Autodesk Inventor part; units mm, degrees
ref_plane "YZ Plane" through (0, 0, 0) normal (1, 0, 0) x (0, 1, 0)
ref_plane "XZ Plane" through (0, 0, 0) normal (0, 1, 0) x (-1, 0, 0)
ref_plane "XY Plane" through (0, 0, 0) normal (0, 0, 1) x (1, 0, 0)
sketch "Sketch1" plane through (0, 0, 0) normal (0, 1, 0) x (-1, 0, 0)
  line L0 (8.5, -37.5) -> (8.5, 37.5) construction
  line L1 (-8.5, 37.5) -> (-8.5, -37.5) construction
  line L2 (15.5, 33) -> (15.5, -33)
  line L3 (-15.5, -33) -> (-15.5, 33) construction
  line L4 (15.5, -33) -> (-15.5, -33)
  line L5 (-8.5, -37.5) -> (8.5, -37.5) construction
  circle A0 centre (8.5, -37.5) radius 2.25
  line L6 (0, -37.5) -> (-8.5, -37.5) construction
  circle A1 centre (-8.5, -37.5) radius 2.25
  line L7 (-15.5, 33) -> (15.5, 33)
  circle A2 centre (-8.5, 37.5) radius 2.25
  line L8 (8.5, 37.5) -> (-8.5, 37.5) construction
  circle A3 centre (8.5, 37.5) radius 2.25
  line L9 (-15.5, -33) -> (15.5, 33) construction
  line L10 (0, 33) -> (0, 19.5) construction
  line L11 (0, 0) -> (15.5, 0) construction
  line L12 (0, 19.5) -> (-39.9, 19.5) construction
  line L13 (-54.9, -40.5) -> (-24.9, -40.5) construction
  circle A4 centre (-54.9, -40.5) radius 2.5
  circle A5 centre (-24.9, -40.5) radius 2.5
  line L14 (-24.9, -40.5) -> (-24.9, -50.5) construction
  line L15 (25.1, 50.5) -> (25.1, -50.5)
  line L16 (25.1, -50.5) -> (-24.9, -50.5)
  line L17 (-15.5, -33) -> (-64.9, -33)
  line L18 (-64.9, -50.5) -> (-24.9, -50.5)
  line L19 (0, 0) -> (-54.9, 0) construction
  line L20 (-54.9, 40.5) -> (-24.9, 40.5) construction
  circle A6 centre (-54.9, 40.5) radius 2.5
  circle A7 centre (-24.9, 40.5) radius 2.5
  line L21 (-24.9, 40.5) -> (-24.9, 50.5) construction
  line L22 (-15.5, 33) -> (-64.9, 33)
  line L23 (-64.9, 50.5) -> (25.1, 50.5)
  line L24 (-24.9, 40.5) -> (-54.9, -40.5)
  circle A8 centre (-39.9, 19.5) radius 3.9303 construction
  line L25 (-15.5, -50.5) -> (-15.5, -33)
  line L26 (-15.5, 33) -> (-15.5, 50.5)
  line L27 (-64.9, -50.5) -> (-64.9, -33)
  line L28 (-64.9, 33) -> (-64.9, 50.5)
  point P0 (0, 0)
  point P1 (8.5, 33)
  dimension "d0" = 8.5
  dimension "d1" = 4.5
  dimension "d2" = 17
  dimension "d3" = 75
  dimension "d4" = 31
  dimension "d9" = 13.5
  dimension "d13" = 39.9
  dimension "d14" = 30
  dimension "d18" = 10
extrude "Extrusion1" add sketch "Sketch1" along normal blind 5 contours L7 L26 L23 L15 L16 L25 L4 L2
extrude "Extrusion2" add sketch "Sketch1" along normal blind 20 contours L22 L28 L23 L26 | L25 L16 L18 L27 L17
properties part number "Servo_fix"
Geometry: final body of the model. Coordinates: model frame, mm. A direction names the side the tool comes from. Give positions to 0.01 mm unless a question says otherwise; leave off trailing zeros. Loops run counter-clockwise (first coordinate to the right, second up) from the corner with the lowest first, then second, coordinate; pieces in that order, holes last. Notation, with made-up numbers: (45.5, -3) -> (82.5, -3) arc R21 cw to (82.5, 11) -> close; hole circle Ø4 at (-36.5, -37.5). An arc over 180 degrees is marked (long way). Put each result on its own line as item: value.
1. Cut plane C-C (y = 3). Count the separate pieces of the cut face and the enclosed holes in it, plus the area to 3 significant figures.
Taken from the geometry:
separate pieces: 1
enclosed holes: 8
area: 3,640 mm2
2. Set-up query: faces 4 (the flat face through (-18, 5, 12)), 5 (the flat face through (64.9, 10, -42)), 6 (the flat face through (33, 8, -33)). Return all of +Z, -Z, +X, -X, +Y, -Y with unobstructed straight access to the full face (end or side cutting, diameter ignored); none if empty.
Taken from the geometry:
face 4: +Z, -Z, -X, +Y
face 5: +Z, -Z, +X, +Y, -Y
face 6: +X, +Y, -Y
3. Cut plane A-A (y = 8.25). Return the cut outline in (x, z).
Taken from the geometry:
outline: (15.5, -50.5) -> (64.9, -50.5) -> (64.9, -33) -> (15.5, -33) -> close; (15.5, 33) -> (64.9, 33) -> (64.9, 50.5) -> (15.5, 50.5) -> close; hole circle Ø5 at (24.9, -40.5); hole circle Ø5 at (24.9, 40.5); hole circle Ø5 at (54.9, -40.5); hole circle Ø5 at (54.9, 40.5)
4. Ray query, line 1 along Z through (x, y) = (54.9, 12); line 2 along Z through (x, y) = (15, 3.5); line 3 along Z through (x, y) = (8.5, 3.6). Return the intervals inside material, ascending. Write a range as [from, to].
Taken from the geometry:
line 1: z = [-50.5, -43], [-38, -33], [33, 38], [43, 50.5]
line 2: z = [-50.5, -33], [33, 50.5]
line 3: z = [-50.5, -39.75], [-35.25, -33], [33, 35.25], [39.75, 50.5]
5. Cut plane B-B (x = -8.5). Return the cut outline in (y, z), plus the area to 3 significant figures.
Taken from the geometry:
outline: (0, -50.5) -> (5, -50.5) -> (5, -39.75) -> (0, -39.75) -> close; (0, -35.25) -> (5, -35.25) -> (5, -33) -> (0, -33) -> close; (0, 33) -> (5, 33) -> (5, 35.25) -> (0, 35.25) -> close; (0, 39.75) -> (5, 39.75) -> (5, 50.5) -> (0, 50.5) -> close
area: 130 mm2
6. Pin query (flat end, axial travel): P1, Ø3, axis at y = 5.5, z = -25.5, coming from the +X side; P2, Ø7.5, axis at y = 14, z = -40.5, coming from the -X side; P3, Ø5, axis at x = -8.5, z = 37.5, coming from the +Y side; P4, Ø3, axis at x = 24.9, z = -40.5, coming from the -Y side. Return the tip coordinate at first contact, or that it passes through.
Taken from the geometry:
P1: stops at x = -15.5
P2: stops at x = 15.5
P3: stops at y = 5
P4: passes through
7. Pull-direction query (Z, two-part tool) for faces 1 (the flat face through (31, 8, 50.5)), 2 (the cylindrical face through (8.79, 2.46, 35.27)), 3 (the flat face through (64.9, 10, 42)); classes: released by +Z, released by -Z, zero draft, split by the parting line, or undercut.
Taken from the geometry:
face 1: released by +Z
face 2: undercut
face 3: zero draft
8. Cut plane D-D (x = 38.5). Return the cut outline in (y, z), plus the area to 3 significant figures.
Taken from the geometry:
outline: (0, -50.5) -> (20, -50.5) -> (20, -33) -> (0, -33) -> close; (0, 33) -> (20, 33) -> (20, 50.5) -> (0, 50.5) -> close
area: 700 mm2
